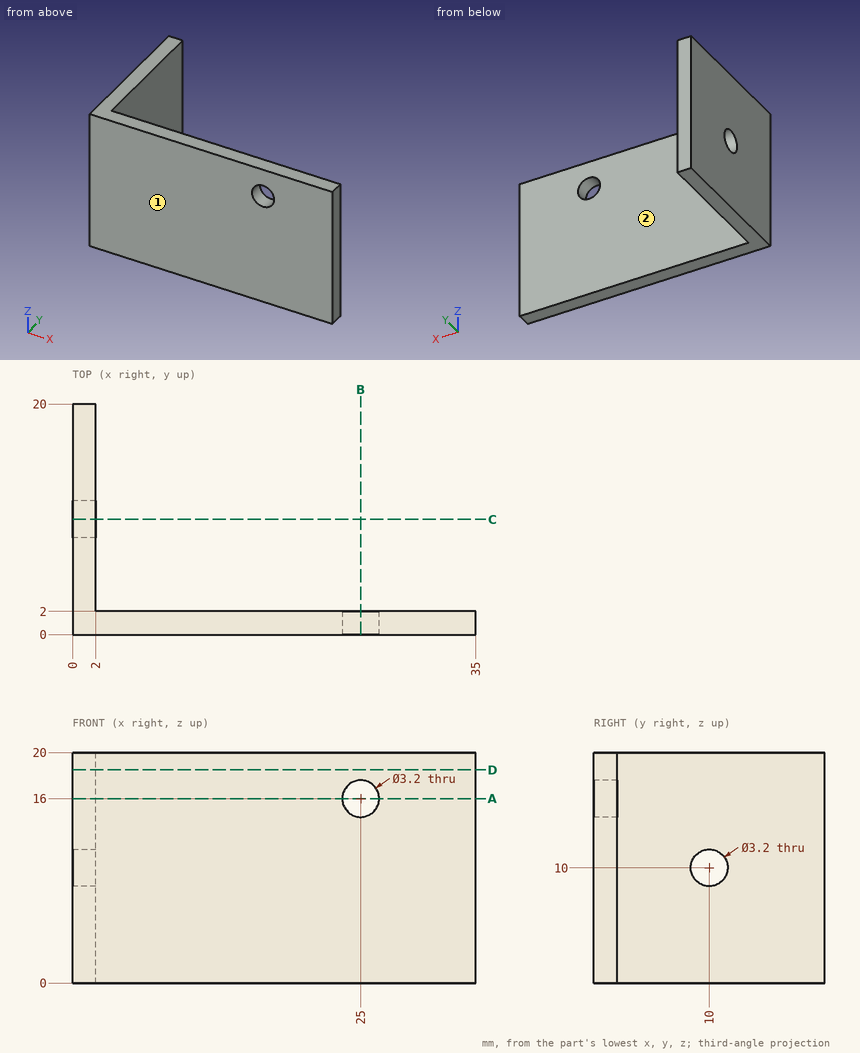
Print and shaded views of the part. All mm, measured from the part's lowest x, y and z. A direction names the side the tool comes from. Give positions to 0.01 mm unless a question says otherwise; leave off trailing zeros. Loops run counter-clockwise (first coordinate to the right, second up) from the corner with the lowest first, then second, coordinate; pieces in that order, holes last. Notation, with made-up numbers: (70.25, -26.5) -> (111.25, -26.5) arc R19 cw to (111.25, -22.5) -> close; hole circle Ø2 at (-20, 71). An arc over 180 degrees is marked (long way). Answer in a Markdown table with one row per item.
Item 1: Slice it at A-A on z = 16. Write the cut outline in (x, y), plus the area to 3 significant figures.
Findings below:
| item | result |
|---|---|
| outline | (0, 0) -> (23.4, 0) -> (23.4, 2) -> (2, 2) -> (2, 20) -> (0, 20) -> close; (26.6, 0) -> (35, 0) -> (35, 2) -> (26.6, 2) -> close |
| area | 99.6 mm² |
Item 2: Slice it at D-D on z = 18.5. Write the cut outline in (x, y), plus the area to 3 significant figures.
Findings below:
| item | result |
|---|---|
| outline | (0, 0) -> (35, 0) -> (35, 2) -> (2, 2) -> (2, 20) -> (0, 20) -> close |
| area | 106 mm² |
Item 3: Slice it at B-B on x = 25. Write the cut outline in (y, z).
Findings below:
| item | result |
|---|---|
| outline | (0, 0) -> (2, 0) -> (2, 14.4) -> (0, 14.4) -> close; (0, 17.6) -> (2, 17.6) -> (2, 20) -> (0, 20) -> close |
Item 4: Probe line 1 along Y through (x, z) = (0.55, 10); line 2 along Z through (x, y) = (25, 1.5); line 3 along Y through (x, z) = (7.5, 4.5). List the from-to ranges inside material, lowest first. Write a range as [from, to].
Findings below:
| item | result |
|---|---|
| line 1 | y = [0, 8.4], [11.6, 20] |
| line 2 | z = [0, 14.4], [17.6, 20] |
| line 3 | y = [0, 2] |
Item 5: Tool access for the marked faces 1 and 2: list every direction of +Z, -Z, +X, -X, +Y, -Y with a clear straight run to the whole face (end or side of a thin tool).
Findings below:
| item | result |
|---|---|
| face 1 | +Z, -Z, +X, -X, -Y |
| face 2 | +Z, -Z, +X, +Y |
Item 6: Slice it at C-C on y = 10. Write the cut outline in (x, z).
Findings below:
| item | result |
|---|---|
| outline | (0, 0) -> (2, 0) -> (2, 8.4) -> (0, 8.4) -> close; (0, 11.6) -> (2, 11.6) -> (2, 20) -> (0, 20) -> close |
Item 7: Flat gauge pins, fed straight in: P1, Ø12, axis at x = 31, z = 13, coming from the +Y side; P2, Ø9, axis at y = 8.5, z = 7, coming from the +X side; P3, Ø1.9, axis at x = 25, z = 16, coming from the +Y side. Where does each tip first touch, or does it go through?
Findings below:
| item | result |
|---|---|
| P1 | stops at y = 2 |
| P2 | stops at x = 2 |
| P3 | passes through |
